Study the drawing (mm; zero at the part's minimum x, y, z) and answer. Round coordinates to 2 decimals unless told otherwise and drop trailing zeros. Loops run counter-clockwise (first coordinate to the right, second up) from the corner with the lowest first, then second, coordinate; pieces in that order, holes last. Notation, with made-up numbers: (8.5, 48.5) -> (54.5, 48.5) arc R6 cw to (54.5, 52.5) -> close; hole circle Ø3 at (61, 39.25). An arc over 180 degrees is marked (long way). Answer in a Markdown table with one row per item. Add a question column.
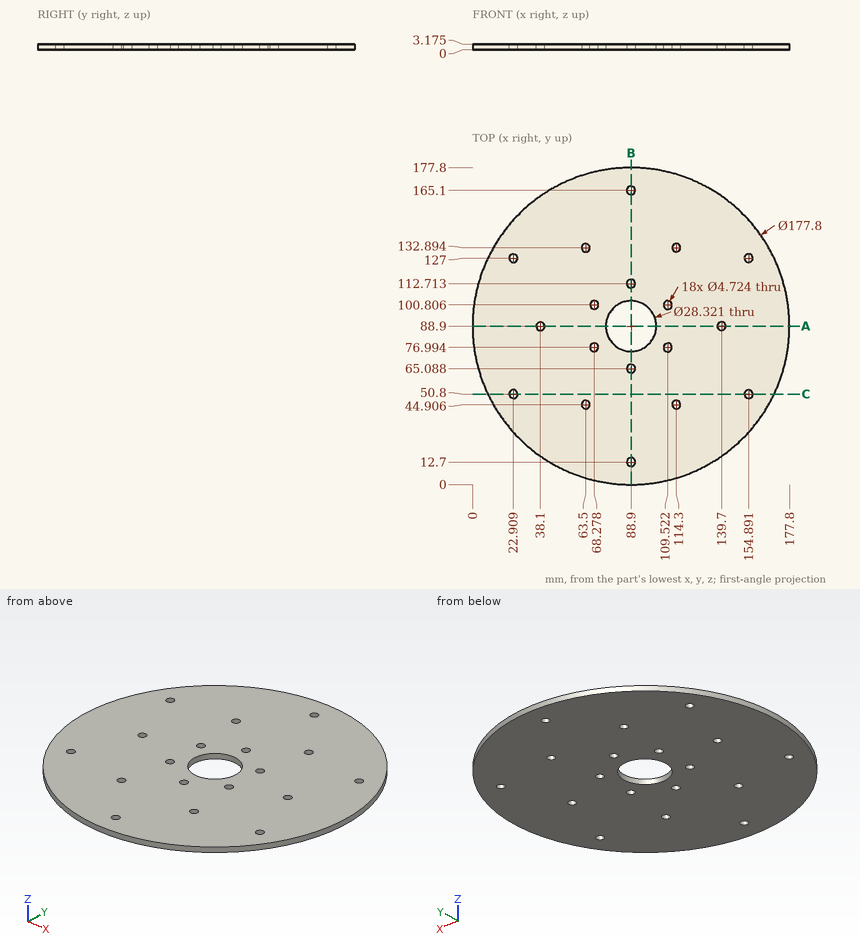
Item 1: A flat-ended cylindrical pin translates along its axis: P1, Ø3, axis at x = 139.7, y = 88.9, coming from the -Z side. Find the tip coordinate at first contact, or state that the pin passes through.
Item 2: Section C-C, the plane y = 50.8 is taken. Write down the section's boundary in (x, z) (1 decimal), and give its area (3 significant figures).
Item 3: Section B-B, the plane x = 88.9 is taken. Give the number of separate pieces and of enclosed holes in the cut face.
Item 4: Consider L1, parallel to X at y = 126, z = 0.6; L2, parallel to X at y = 77.5, z = 3.05 (1 decimal); L3, parallel to X at y = 43, z = 0.9 (1 decimal). Determine where each line is inside the solid, lowest interval first. Write a range as from..to.
Item 5: Section A-A, the plane y = 88.9 is taken. Write down the section's boundary in (x, z) (1 decimal).
Here are the results:
| question | item | result |
|---|---|---|
| 1 | P1 | passes through |
| 2 | outline | (8.6, 0) -> (20.5, 0) -> (20.5, 3.2) -> (8.6, 3.2) -> close; (25.3, 0) -> (152.5, 0) -> (152.5, 3.2) -> (25.3, 3.2) -> close; (157.3, 0) -> (169.2, 0) -> (169.2, 3.2) -> (157.3, 3.2) -> close |
| 2 | area | 480 mm² |
| 3 | separate pieces | 6 |
| 3 | enclosed holes | 0 |
| 4 | L1 | x = 8.11..20.77, 25.05..152.75, 157.03..169.69 |
| 4 | L2 | x = 0.7..66, 70.6..80.5, 97.3..107.2, 111.8..177.1 |
| 4 | L3 | x = 12.8..62.1, 64.9..112.9, 115.7..165 |
| 5 | outline | (0, 0) -> (35.7, 0) -> (35.7, 3.2) -> (0, 3.2) -> close; (40.5, 0) -> (74.7, 0) -> (74.7, 3.2) -> (40.5, 3.2) -> close; (103.1, 0) -> (137.3, 0) -> (137.3, 3.2) -> (103.1, 3.2) -> close; (142.1, 0) -> (177.8, 0) -> (177.8, 3.2) -> (142.1, 3.2) -> close |
